```python
from build123d import *

# Parameters (mm, degrees)
SKETCH1_W             = 222.25
SKETCH1_H             = 114.3
SKETCH1_R             = 50.8
BOSS_EXTRUDE1_DEPTH   = 2.54
BOSS_EXTRUDE2_DEPTH   = 222.25
SKETCH4_W             = 222.25
SKETCH4_H             = 9.525
BOSS_EXTRUDE3_DEPTH   = 9.017
F_6_32_TAPPED_HOLE1_D = 2.7051
LPATTERN1_COUNT       = 18
LPATTERN1_PITCH       = 12.7
FILLET1_R             = 3.175


with BuildPart() as part:
    # Sketch1 → Boss-Extrude1 (new body)
    with BuildSketch(Plane.XY):
        with Locations((57.15, 0)):
            Rectangle(SKETCH1_W, SKETCH1_H)
        Circle(SKETCH1_R, mode=Mode.SUBTRACT)
    extrude(amount=BOSS_EXTRUDE1_DEPTH)

    # Sketch3 → Boss-Extrude2 (add)
    with BuildSketch(Plane(origin=(168.275, 0, 0), x_dir=(0, 0, -1), z_dir=(1, 0, 0))):
        Polygon((-2.54, 57.15), (-9.017, 57.15), (-9.017, 50.8), (-5.842, 50.8), (-5.842, 53.975), (-2.54, 53.975), align=None)
    boss_extrude2 = extrude(amount=-BOSS_EXTRUDE2_DEPTH)

    # Mirror1: Boss-Extrude2 across plane
    add(boss_extrude2.mirror(Plane(origin=(0, 0, 0), x_dir=(0, 0, 1), z_dir=(0, -1, 0))))

    # Sketch4 → Boss-Extrude3 (add)
    with BuildSketch(Plane.XY):
        with Locations((57.15, -61.9125)):
            Rectangle(SKETCH4_W, SKETCH4_H)
        with Locations((57.15, 61.9125)):
            Rectangle(SKETCH4_W, SKETCH4_H)
    extrude(amount=BOSS_EXTRUDE3_DEPTH)

    # #6-32 Tapped Hole1 (through all)
    with Locations(Plane.XY.offset(9.017)):
        with Locations((-50.8, -61.595), (-50.8, 61.595)):
            f_6_32_tapped_hole1 = Hole(F_6_32_TAPPED_HOLE1_D / 2)

    # LPattern1: #6-32 Tapped Hole1 ×18
    with Locations(*[(i * LPATTERN1_PITCH, 0, 0) for i in range(1, LPATTERN1_COUNT)]):
        add(f_6_32_tapped_hole1, mode=Mode.SUBTRACT)

    # Fillet1
    fillet1_edges = [part.edges().sort_by_distance(p)[0] for p in [
        (57.15, 53.975, 5.842),
        (57.15, -53.975, 5.842),
    ]]
    fillet(fillet1_edges, radius=FILLET1_R - 0.0001)  # a hair under: the kernel refuses the full size


solid = part.part
```
Here's how the part is built. I have some questions about the finished solid (model axes, mm). Give positions to 0.01 mm unless a question says otherwise; leave off trailing zeros. Loops run counter-clockwise (first coordinate to the right, second up) from the corner with the lowest first, then second, coordinate; pieces in that order, holes last. Notation, with made-up numbers: (81.5, -34) -> (90.5, -34) arc R12 cw to (90.5, -22) -> close; hole circle Ø10 at (-9.75, 2). An arc over 180 degrees is marked (long way). Use one line per item in the form item = value. Start each with the question number.
1) For P1, Ø3.5, axis at x = 38.1, y = 61.595, coming from the -Z side; P2, Ø2, axis at x = 152.4, y = -61.595, coming from the -Z side; P3, Ø10, axis at x = 112.5, y = 44.5, coming from the +Z side, each with a flat end and sliding along its axis, tell me the tip position at first contact or that it passes through.
2) Thinking about a two-plate mould opening in Y: for faces 1 (the face through (168.275, -1, 2)), 2 (the face through (56, -66.675, 4)), 3 (the face through (-11.012, -49.592, 1.252)), which applies, +Y half, -Y half, draft (parallel to the pull), parting line (faces both ways), or undercut?
3) Please list where these lines run through material, in increasing order: line 1 along Y through (x, z) = (0, 1.65) (3 decimals); line 2 along Y through (x, z) = (47, 8.5) (3 decimals); line 3 along Y through (x, z) = (-25, 5.5) (3 decimals).
4) Imagine slicing it at C-C (y = 3). Please give me the cut outline in (x, z) (3 decimals), then the cut area to 3 significant figures.
5) Imagine slicing it at A-A (y = -32.5). Please give me the cut outline in (x, z) (3 decimals).
Check values:
q1.P1 = 0
q1.P2 = through
q1.P3 = 2.54
q2.face_1 = draft
q2.face_2 = -Y half
q2.face_3 = undercut
q3.line_1 = -66.675 to -62.948, -60.242 to -50.8, 50.8 to 60.242, 62.948 to 66.675
q3.line_2 = -66.675 to -50.8, 50.8 to 66.675
q3.line_3 = -66.675 to -62.887, -60.303 to -52.234, 52.234 to 60.303, 62.887 to 66.675
q4.outline = (-53.975, 0) -> (-50.711, 0) -> (-50.711, 2.54) -> (-53.975, 2.54) -> close; (50.711, 0) -> (168.275, 0) -> (168.275, 2.54) -> (50.711, 2.54) -> close
q4.area = 307 mm^2
q5.outline = (-53.975, 0) -> (-39.043, 0) -> (-39.043, 2.54) -> (-53.975, 2.54) -> close; (39.043, 0) -> (168.275, 0) -> (168.275, 2.54) -> (39.043, 2.54) -> close
